Part model, mm, in its own coordinate system. Face numbers are marked on the shaded views. A direction names the side the tool comes from. Give positions to 0.01 mm unless a question says otherwise; leave off trailing zeros. Write each loop counter-clockwise with the first axis right and the second up, starting at its lowest first coordinate (ties: lowest second). Pieces come first, ordered by that corner, then holes.
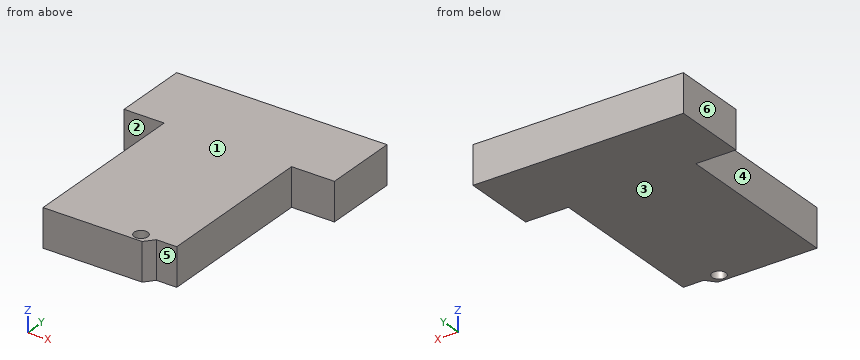
```python
from build123d import *

# Parameters (mm, degrees)
BOSS_EXTRUDE1_DEPTH = 12.7
SKETCH1_9_W         = 14.260820695
SKETCH1_9_H         = 54.5
SKETCH1_9_R         = 2.277625676
CUT_EXTRUDE6_DEPTH  = 12.7


with BuildPart() as part:
    # Sketch1 → Boss-Extrude1 (new body)
    with BuildSketch(Plane.XY):
        Polygon((-70, 3.04), (-59.19389142, 3.04), (-56.643028541, 0), (-23.643028541, 0), (-21.092165662, 3.04), (0, 3.04), (0, 82.5), (-70, 82.5), align=None)
    extrude(amount=BOSS_EXTRUDE1_DEPTH)

    # Sketch1<9> → Cut-Extrude6 (cut)
    with BuildSketch(Plane.XY):
        Polygon((-70, 57.54), (-70, 3.04), (-59.19389142, 3.04), (-56.643028541, 0), (-56.643028541, 57.54), align=None)
        with Locations((-7.130410348, 30.29)):
            Rectangle(SKETCH1_9_W, SKETCH1_9_H)
        with Locations((-26.17389142, 3.04)):
            Circle(SKETCH1_9_R)
    extrude(amount=CUT_EXTRUDE6_DEPTH, mode=Mode.SUBTRACT)


solid = part.part
```
1) 3-axis set-ups, long thin cutter, end or side, ignore diameter. For the marked faces 4, 5 and 6: which of +Z, -Z, +X, -X, +Y, -Y reach the whole face in a straight line?
Answers follow:
face 4: +Z, -Z, -X, -Y
face 5: +Z, -Z, +X, -Y
face 6: +Z, -Z, -X, +Y, -Y
2) Pin check, flat tips, straight feed: pin 1 Ø3 at (y, z) = (51.5, 7) entering from +X; pin 2 Ø2.5 at (x, y) = (-26.17, 3.04) entering from +Z; pin 3 Ø6 at (y, z) = (31, 2.5) entering from -X; pin 4 Ø2 at (x, z) = (-18, 7) entering from -Y. Stop position of each tip, or through.
Answers follow:
pin 1: stops at x = -14.26
pin 2: passes through
pin 3: stops at x = -56.64
pin 4: stops at y = 3.04
3) Saw through at B-B, the plane y = 27. Write the cut outline in (x, z), then the cut area to 3 significant figures.
Answers follow:
outline: (-56.64, 0) - (-14.26, 0) - (-14.26, 12.7) - (-56.64, 12.7) - close
area: 538 mm2
4) Two-plate mould, pull along Z, no slides. Class the marked faces 1, 2 and 3: +Z half, -Z half, draft (parallel to the pull), parting line (faces both ways), or undercut.
Answers follow:
face 1: +Z half
face 2: draft
face 3: -Z half
5) Saw through at C-C, the plane x = -60. Write the cut outline in (y, z).
Answers follow:
outline: (57.54, 0) - (82.5, 0) - (82.5, 12.7) - (57.54, 12.7) - close
6) Wall check: L1, parallel to X at y = 57, z = 8.5; L2, parallel to Y at x = -24.5, z = 3.25; L3, parallel to Y at x = -12, z = 4. Give the ranges that are in metal, low to high.
Answers follow:
L1: x = -56.64 to -14.26
L2: y = 0 to 1.5, 4.58 to 82.5
L3: y = 57.54 to 82.5
7) Saw through at A-A, the plane z = 10.25. Write the cut outline in (x, y).
Answers follow:
outline: (-70, 57.54) - (-56.64, 57.54) - (-56.64, 0) - (-23.64, 0) - (-21.09, 3.04) - (-14.26, 3.04) - (-14.26, 57.54) - (0, 57.54) - (0, 82.5) - (-70, 82.5) - close; hole circle Ø4.56 at (-26.17, 3.04)
